Autodesk Inventor part; units mm, degrees
ref_plane "YZ Plane" through (0, 0, 0) normal (1, 0, 0) x (0, 1, 0)
ref_plane "XZ Plane" through (0, 0, 0) normal (0, 1, 0) x (-1, 0, 0)
ref_plane "XY Plane" through (0, 0, 0) normal (0, 0, 1) x (1, 0, 0)
sketch "Sketch1" plane through (0, 0, 0) normal (0, 1, 0) x (-1, 0, 0)
  circle A0 centre (0.6852, 198.77) radius 2.1844
  circle A1 centre (13.3852, 198.77) radius 2.1844
  circle A2 centre (13.3833, -182.23) radius 2.1844
  circle A3 centre (0.6833, -182.2338) radius 2.1844
  arc A4 (19.7352, 198.77) -> (13.3852, 205.12) centre (13.3852, 198.77) ccw
  arc A5 (0.6852, 205.12) -> (-5.0541, 201.487) centre (0.6852, 198.77) ccw
  arc A6 (13.3795, -188.5838) -> (19.7372, -182.23) centre (13.3833, -182.23) ccw
  arc A7 (-5.0525, -184.9492) -> (0.6814, -188.5799) centre (0.6833, -182.2338) ccw
  line L0 (13.3852, 205.12) -> (0.6852, 205.12)
  line L1 (13.3833, -188.5838) -> (0.6814, -188.5799)
  line L2 (19.7352, 198.77) -> (19.7372, -182.23)
  line L3 (-18.3648, 173.37) -> (-18.3648, -156.83)
  line L4 (-18.3648, -156.83) -> (-5.0525, -184.9492)
  line L5 (-18.3648, 173.37) -> (-5.0541, 201.487)
  point P0 (0, 0)
  dimension "d0" = 330.2
extrude "Extrusion1" add sketch "Sketch1" along normal blind 1.5875
properties part number "skirt" material "Acetal Resin, White"
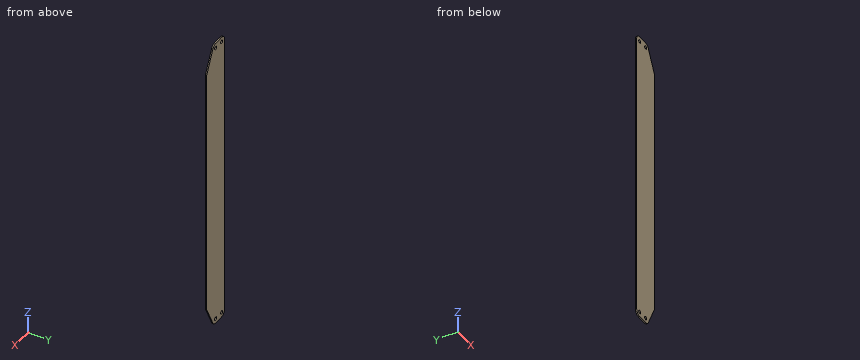
Read the model definition and answer for the solid it produces. Units are mm, in the model's axes. Coordinates: 2 decimals unless noted, no trailing zeros. Order: outer loops, then holes, each group sorted by start corner. A loop starts at its lowest first (then second) coordinate and runs counter-clockwise, first axis right, second up. Notation, with made-up numbers: M -37.5,-27.75 L -0.5,-27.75 A22 ccw -0.5,2.25 Z; hole C 63.25,1.5 d3. An arc over 180 degrees is marked long. Put each result on its own line as item: value. Start each with the question number.
Item 1: Consider probe 1 along Z at (x, y) = (-1, 1.3); probe 2 along Z at (x, y) = (0, 0.65); probe 3 along X at (y, z) = (0.7, -182.23). Determine where each line is inside the solid, lowest interval first. Write a range as [from, to].
Item 2: Section B-B, the plane x = 14.5 is taken. Determine the outline of the cut face in (y, z).
Item 3: Given pin 1 Ø4 at (x, z) = (-0.69, 198.77) entering from -Y, flat-ended and moving along its own axis, determine where the tip first touches the part or whether it passes through.
Item 4: Section A-A, the plane y = 0.7 is taken. Determine the outline of the cut face in (x, z).
Computed:
1. probe 1: z = [-188.58, -184.4], [-180.07, 196.61], [200.93, 205.12]
1. probe 2: z = [-188.54, -184.31], [-180.16, 196.7], [200.84, 205.08]
1. probe 3: x = [-19.74, -15.57], [-11.2, -2.87], [1.5, 6.34]
2. outline: M 0,-164.99 L 1.59,-164.99 L 1.59,181.53 L 0,181.53 Z
3. pin 1: passes through
4. outline: M -19.74,-182.23 A6.35 ccw -13.38,-188.58 L -0.68,-188.58 A6.35 ccw 5.05,-184.95 L 18.36,-156.83 L 18.36,173.37 L 5.05,201.49 A6.35 ccw -0.69,205.12 L -13.39,205.12 A6.35 ccw -19.74,198.77 Z; hole C -13.38,-182.23 d4.37; hole C -13.39,198.77 d4.37; hole C -0.68,-182.23 d4.37; hole C -0.69,198.77 d4.37
